Job drawing, mm, ordinate dimensions from the low corner. One solid piece. Give positions to 0.01 mm unless a question says otherwise; leave off trailing zeros. Order: outer loops, then holes, each group sorted by start corner. A loop starts at its lowest first (then second) coordinate and runs counter-clockwise, first axis right, second up.
1. Slice it at B-B on y = 1.25. List the corners of the cut face in (x, z).
2. Slice it at A-A on x = 37. List the corners of the cut face in (y, z), and give its area (3 significant figures).
3. Drop a flat-ended pin along its axis: pin 1 Ø6 at (x, y) = (27, 8) entering from +Z. Give the stop position or say it passes through.
4. Mould opens along X. For the marked faces 1 and 2 say: +X half, -X half, draft (parallel to the pull), parting line (faces both ways), or undercut.
5. Probe line 1 (Z direction, x = 33.5, y = 8.5); line 2 (X direction, y = 5, z = 2.4); line 3 (X direction, y = 3, z = 2.6) (1 decimal). List the from-to ranges inside material, lowest first.
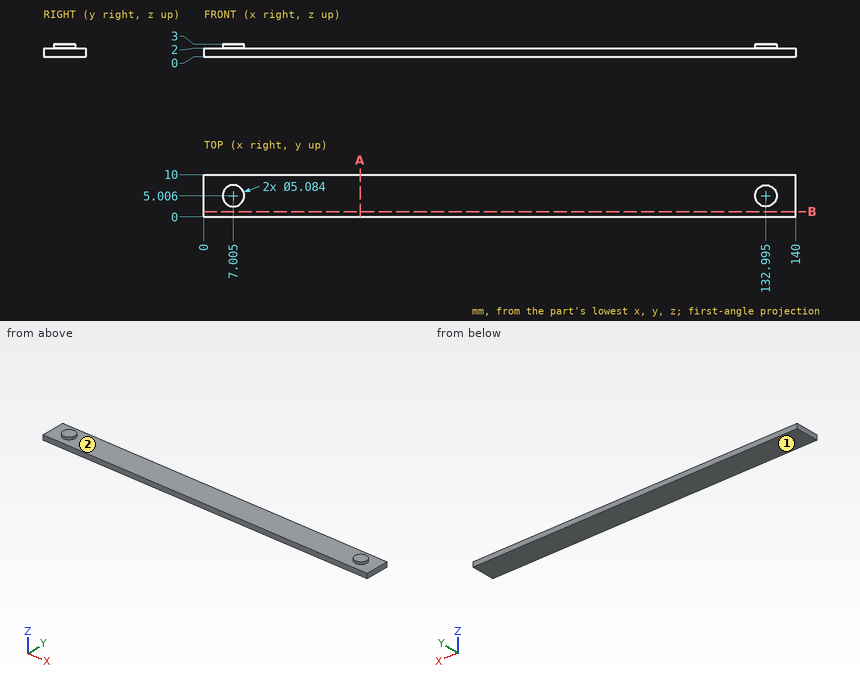
Data:
1. outline: (0, 0) - (140, 0) - (140, 2) - (0, 2) - close
2. outline: (0, 0) - (10, 0) - (10, 2) - (0, 2) - close
2. area: 20.0 mm2
3. pin 1: stops at z = 2
4. face 1: draft
4. face 2: undercut
5. line 1: z = 0 to 2
5. line 2: x = 4.46 to 9.55, 130.45 to 135.54
5. line 3: x = 5.4 to 8.6, 131.4 to 134.6
